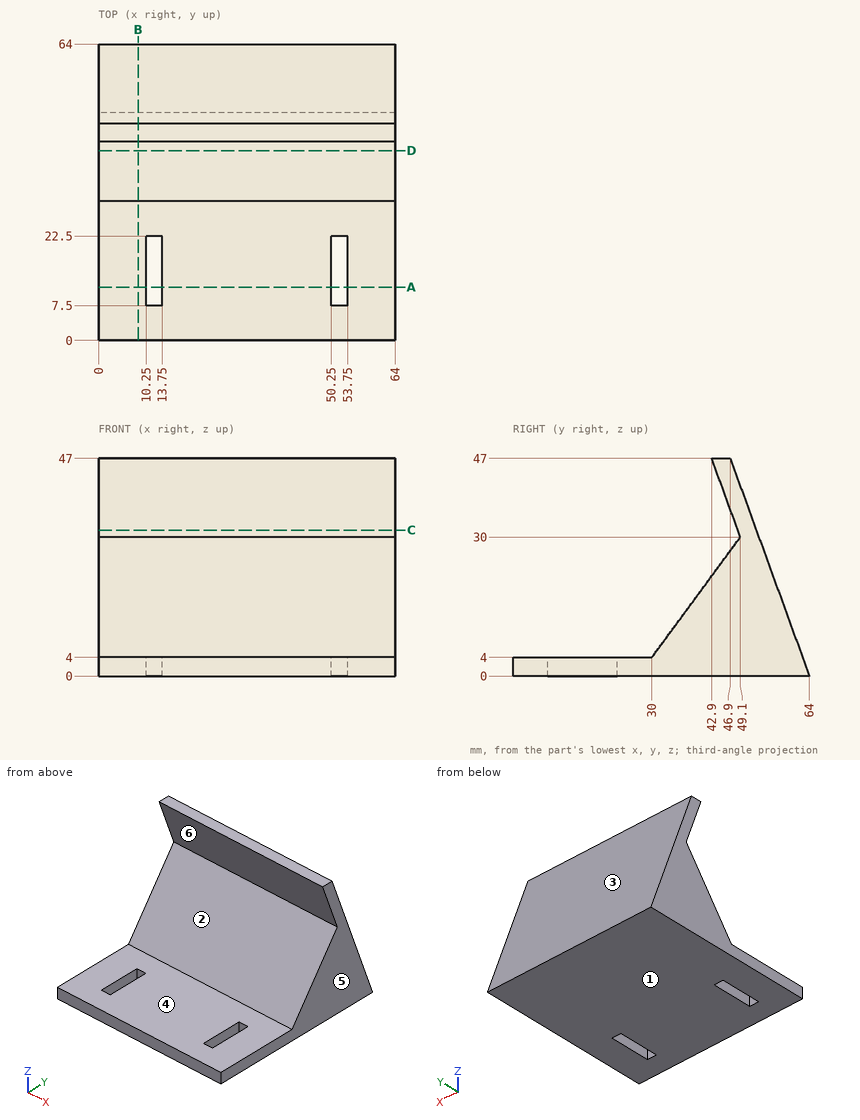
Print and shaded views of the part. All mm, measured from the part's lowest x, y and z. A direction names the side the tool comes from. Give positions to 0.01 mm unless a question says otherwise; leave off trailing zeros. Order: outer loops, then holes, each group sorted by start corner. A loop starts at its lowest first (then second) coordinate and runs counter-clockwise, first axis right, second up. Notation, with made-up numbers: (-30.75, -10) -> (-16.75, -10) arc R15 cw to (-16.75, 16) -> close; hole circle Ø2 at (4.5, -24). An arc over 180 degrees is marked (long way). Use CSV: the item, a comma, the result in double quotes.
1. Band-saw the part on B-B, the plane x = 8.5. Give the cut face in (y, z).
Outcome:
outline,"(0, 0) -> (64, 0) -> (46.9, 47) -> (42.9, 47) -> (49.1, 30) -> (30, 4) -> (0, 4) -> close"
2. Mould opens along Z. For the marked faces 1, 2 and 3 say: +Z half, -Z half, draft (parallel to the pull), parting line (faces both ways), or undercut.
Outcome:
face 1,"-Z half"
face 2,"undercut"
face 3,"+Z half"
3. Band-saw the part on A-A, the plane y = 11.5. Give the cut face in (x, z).
Outcome:
outline,"(0, 0) -> (10.25, 0) -> (10.25, 4) -> (0, 4) -> close; (13.75, 0) -> (50.25, 0) -> (50.25, 4) -> (13.75, 4) -> close; (53.75, 0) -> (64, 0) -> (64, 4) -> (53.75, 4) -> close"
4. Drill centre lines: line 1 along Z through (x, y) = (46, 4); line 2 along Y through (x, z) = (25.5, 37); line 3 along Z through (x, y) = (26, 42). Where is each one in solid material? Low to high. Write a range as from..to.
Outcome:
line 1,"0..4"
line 2,"46.55..50.54"
line 3,"0..20.34"
5. Drop flat-ended pins along their axis: pin 1 (1 mm diameter, centred on x = 53, z = 2, fed in from +Y); pin 2 (6 mm diameter, centred on x = 54.5, z = 39, fed in from +Y); pin 3 (2 mm diameter, centred on x = 32, z = 9, fed in from +Y). Give the stop position or say it passes through.
Outcome:
pin 1,"y = 63.45"
pin 2,"y = 50.9"
pin 3,"y = 61.09"
6. 3-axis set-ups, long thin cutter, end or side, ignore diameter. For the marked faces 4, 5 and 6: which of +Z, -Z, +X, -X, +Y, -Y reach the whole face in a straight line?
Outcome:
face 4,"+Z, +X, -X, -Y"
face 5,"+Z, -Z, +X, +Y, -Y"
face 6,"+X, -X, -Y"
7. Band-saw the part on C-C, the plane z = 31.5. Give the cut face in (x, y), then the cut area to 3 significant figures.
Outcome:
outline,"(0, 48.55) -> (64, 48.55) -> (64, 52.54) -> (0, 52.54) -> close"
area,"255 mm²"
8. Band-saw the part on D-D, the plane y = 41. Give the cut face in (x, z).
Outcome:
outline,"(0, 0) -> (64, 0) -> (64, 18.97) -> (0, 18.97) -> close"
